Build history of the part. All positions in model axes, mm. Round coordinates to 2 decimals unless told otherwise and drop trailing zeros. Loops run counter-clockwise (first coordinate to the right, second up) from the corner with the lowest first, then second, coordinate; pieces in that order, holes last. Notation, with made-up numbers: M 13.5,-9 L 68.5,-9 A18 cw 68.5,-5 Z; hole C 33,-18.5 d7. An arc over 180 degrees is marked long. One line per item, written item: value.
```python
from build123d import *

# Parameters (mm, degrees)
SKETCH1_R           = 3.5
SKETCH1_W           = 6
SKETCH1_H           = 6
BOSS_EXTRUDE1_DEPTH = 6
CUT_EXTRUDE1_REACH  = 8
SKETCH2_R           = 1.5


with BuildPart() as part:
    # Sketch1 → Boss-Extrude1 (new body)
    with BuildSketch(Plane.XY):
        with BuildLine():
            Line((0, 5.15), (0, 0))
            Line((0, 0), (74, 0))
            Line((74, 0), (74, 5.15))
            Line((74, 5.15), (68, 5.15))
            Line((68, 5.15), (68, 11.15))
            Line((68, 11.15), (74, 11.15))
            Line((74, 11.15), (74, 26.84))
            Line((74, 26.84), (68, 26.84))
            Line((68, 26.84), (68, 32.84))
            Line((68, 32.84), (74, 32.84))
            Line((74, 32.84), (74, 91.26))
            ThreePointArc((74, 91.26), (71.071067812, 98.331067812), (64, 101.26))
            Line((64, 101.26), (10, 101.26))
            ThreePointArc((10, 101.26), (2.928932188, 98.331067812), (0, 91.26))
            Line((0, 91.26), (0, 32.84))
            Line((0, 32.84), (6, 32.84))
            Line((6, 32.84), (6, 26.84))
            Line((6, 26.84), (0, 26.84))
            Line((0, 26.84), (0, 11.15))
            Line((0, 11.15), (6, 11.15))
            Line((6, 11.15), (6, 5.15))
            Line((6, 5.15), (0, 5.15))
        make_face()
        with Locations((12, 10)):
            Circle(SKETCH1_R, mode=Mode.SUBTRACT)
        with Locations((21.81, 29.84)):
            Rectangle(SKETCH1_W, SKETCH1_H, mode=Mode.SUBTRACT)
        with Locations((37, 10)):
            Circle(SKETCH1_R, mode=Mode.SUBTRACT)
        with Locations((62, 10)):
            Circle(SKETCH1_R, mode=Mode.SUBTRACT)
        with Locations((52.19, 29.84)):
            Rectangle(SKETCH1_W, SKETCH1_H, mode=Mode.SUBTRACT)
    extrude(amount=BOSS_EXTRUDE1_DEPTH)

    # Sketch2 → Cut-Extrude1 (cut, up to next)
    with BuildSketch(Plane.XY.offset(6), mode=Mode.PRIVATE) as cut_extrude1_sk1:
        with Locations((3, 15.84)):
            Circle(SKETCH2_R)
    cut_extrude1_tool1 = extrude(cut_extrude1_sk1.sketch, amount=-CUT_EXTRUDE1_REACH, mode=Mode.PRIVATE) & part.part
    add(cut_extrude1_tool1.solids().sort_by_distance((3, 15.84, 6))[0], mode=Mode.SUBTRACT)
    # Sketch2 → Cut-Extrude1 (cut, up to next)
    with BuildSketch(Plane.XY.offset(6), mode=Mode.PRIVATE) as cut_extrude1_sk2:
        with Locations((11.5, 29.84)):
            Circle(SKETCH2_R)
    cut_extrude1_tool2 = extrude(cut_extrude1_sk2.sketch, amount=-CUT_EXTRUDE1_REACH, mode=Mode.PRIVATE) & part.part
    add(cut_extrude1_tool2.solids().sort_by_distance((11.5, 29.84, 6))[0], mode=Mode.SUBTRACT)
    # Sketch2 → Cut-Extrude1 (cut, up to next)
    with BuildSketch(Plane.XY.offset(6), mode=Mode.PRIVATE) as cut_extrude1_sk3:
        with Locations((62.5, 29.84)):
            Circle(SKETCH2_R)
    cut_extrude1_tool3 = extrude(cut_extrude1_sk3.sketch, amount=-CUT_EXTRUDE1_REACH, mode=Mode.PRIVATE) & part.part
    add(cut_extrude1_tool3.solids().sort_by_distance((62.5, 29.84, 6))[0], mode=Mode.SUBTRACT)
    # Sketch2 → Cut-Extrude1 (cut, up to next)
    with BuildSketch(Plane.XY.offset(6), mode=Mode.PRIVATE) as cut_extrude1_sk4:
        with Locations((71, 15.84)):
            Circle(SKETCH2_R)
    cut_extrude1_tool4 = extrude(cut_extrude1_sk4.sketch, amount=-CUT_EXTRUDE1_REACH, mode=Mode.PRIVATE) & part.part
    add(cut_extrude1_tool4.solids().sort_by_distance((71, 15.84, 6))[0], mode=Mode.SUBTRACT)


solid = part.part
```
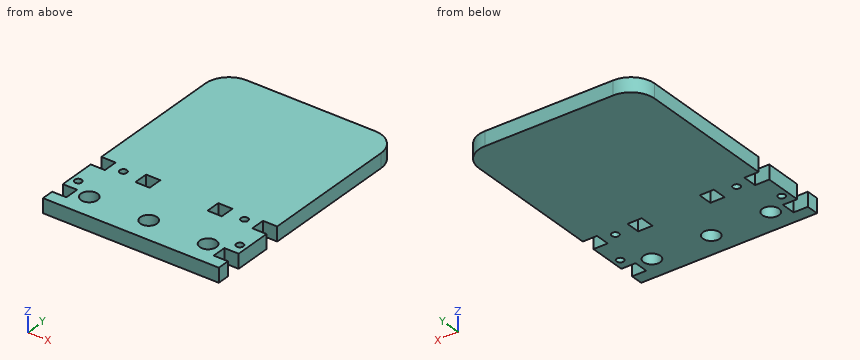
Item 1: Slice it at D-D, the plane z = 4.3. Give the number of separate pieces and of enclosed holes in the cut face, and give its area (3 significant figures).
Check values:
separate pieces: 1
enclosed holes: 9
area: 7,090 mm2
Item 2: Wall check: line 1 along Y through (x, z) = (20, 4.85); line 2 along Y through (x, z) = (11.5, 3); line 3 along Y through (x, z) = (3, 2.9). Give the ranges that are in metal, low to high.
Check values:
line 1: y = 0 to 26.84, 32.84 to 101.26
line 2: y = 0 to 6.54, 13.46 to 28.34, 31.34 to 101.26
line 3: y = 0 to 5.15, 11.15 to 14.34, 17.34 to 26.84, 32.84 to 98.4
Item 3: Slice it at A-A, the plane x = 37. Give the cut face in (y, z), and give its area (3 significant figures).
Check values:
outline: M 0,0 L 6.5,0 L 6.5,6 L 0,6 Z; M 13.5,0 L 101.26,0 L 101.26,6 L 13.5,6 Z
area: 566 mm2
Item 4: Slice it at C-C, the plane y = 10. Give the cut face in (x, z).
Check values:
outline: M 6,0 L 8.5,0 L 8.5,6 L 6,6 Z; M 15.5,0 L 33.5,0 L 33.5,6 L 15.5,6 Z; M 40.5,0 L 58.5,0 L 58.5,6 L 40.5,6 Z; M 65.5,0 L 68,0 L 68,6 L 65.5,6 Z
Item 5: Slice it at B-B, the plane y = 29.84. Give the cut face in (x, z), and give its area (3 significant figures).
Check values:
outline: M 6,0 L 10,0 L 10,6 L 6,6 Z; M 13,0 L 18.81,0 L 18.81,6 L 13,6 Z; M 24.81,0 L 49.19,0 L 49.19,6 L 24.81,6 Z; M 55.19,0 L 61,0 L 61,6 L 55.19,6 Z; M 64,0 L 68,0 L 68,6 L 64,6 Z
area: 264 mm2
Item 6: Drop flat-ended pins along their axis: P1, Ø2, axis at y = 29.5, z = 2, coming from the -X side; P2, Ø2.5, axis at x = 11.5, y = 29.84, coming from the -Z side; P3, Ø1.8, axis at y = 30.5, z = 4.5, coming from the +X side; P4, Ø3, axis at x = 4, z = 3, coming from the +Y side. Give the stop position or say it passes through.
Check values:
P1: stops at x = 6
P2: passes through
P3: stops at x = 68
P4: stops at y = 100.19
